Autodesk Inventor part; units mm, degrees
ref_plane "YZ Plane" through (0, 0, 0) normal (1, 0, 0) x (0, 1, 0)
ref_plane "XZ Plane" through (0, 0, 0) normal (0, 1, 0) x (-1, 0, 0)
ref_plane "XY Plane" through (0, 0, 0) normal (0, 0, 1) x (1, 0, 0)
sketch "C12,5-5, 470uF_126" plane through (0, 0, 0) normal (0, 0, 1) x (1, 0, 0)
  line L0 (0.9403, 6.3386) -> (1.557, 6.216)
  line L1 (1.557, 6.216) -> (2.1588, 6.0334)
  line L2 (2.1588, 6.0334) -> (2.7398, 5.7928)
  line L3 (2.7398, 5.7928) -> (3.2944, 5.4963)
  line L4 (3.2944, 5.4963) -> (3.8172, 5.147)
  line L5 (3.8172, 5.147) -> (4.3033, 4.748)
  line L6 (4.3033, 4.748) -> (4.748, 4.3034)
  line L7 (4.748, 4.3034) -> (5.147, 3.8172)
  line L8 (5.147, 3.8172) -> (5.4963, 3.2944)
  line L9 (5.4963, 3.2944) -> (5.7928, 2.7398)
  line L10 (5.7928, 2.7398) -> (6.0334, 2.1588)
  line L11 (6.0334, 2.1588) -> (6.216, 1.557)
  line L12 (6.216, 1.557) -> (6.3386, 0.9403)
  line L13 (6.3386, 0.9403) -> (6.4003, 0.3144)
  line L14 (6.4003, 0.3144) -> (6.4003, 0)
  line L15 (6.4003, 0) -> (6.4003, -0.3144)
  line L16 (6.4003, -0.3144) -> (6.3386, -0.9403)
  line L17 (6.3386, -0.9403) -> (6.216, -1.557)
  line L18 (6.216, -1.557) -> (6.0334, -2.1588)
  line L19 (6.0334, -2.1588) -> (5.7928, -2.7398)
  line L20 (5.7928, -2.7398) -> (5.4963, -3.2944)
  line L21 (5.4963, -3.2944) -> (5.147, -3.8172)
  line L22 (5.147, -3.8172) -> (4.748, -4.3033)
  line L23 (4.748, -4.3033) -> (4.3033, -4.748)
  line L24 (4.3033, -4.748) -> (3.8172, -5.147)
  line L25 (3.8172, -5.147) -> (3.2944, -5.4963)
  line L26 (3.2944, -5.4963) -> (2.7398, -5.7928)
  line L27 (2.7398, -5.7928) -> (2.1588, -6.0334)
  line L28 (2.1588, -6.0334) -> (1.557, -6.216)
  line L29 (1.557, -6.216) -> (0.9403, -6.3386)
  line L30 (0.9403, -6.3386) -> (0.3144, -6.4003)
  line L31 (0.3144, -6.4003) -> (-0.3144, -6.4003)
  line L32 (-0.3144, -6.4003) -> (-0.9403, -6.3386)
  line L33 (-0.9403, -6.3386) -> (-1.557, -6.216)
  line L34 (-1.557, -6.216) -> (-2.1588, -6.0334)
  line L35 (-2.1588, -6.0334) -> (-2.7398, -5.7928)
  line L36 (-2.7398, -5.7928) -> (-3.2944, -5.4963)
  line L37 (-3.2944, -5.4963) -> (-3.8172, -5.147)
  line L38 (-3.8172, -5.147) -> (-4.3034, -4.748)
  line L39 (-4.3034, -4.748) -> (-4.748, -4.3033)
  line L40 (-4.748, -4.3033) -> (-5.147, -3.8172)
  line L41 (-5.147, -3.8172) -> (-5.4963, -3.2944)
  line L42 (-5.4963, -3.2944) -> (-5.7928, -2.7398)
  line L43 (-5.7928, -2.7398) -> (-6.0334, -2.1588)
  line L44 (-6.0334, -2.1588) -> (-6.216, -1.557)
  line L45 (-6.216, -1.557) -> (-6.3386, -0.9403)
  line L46 (-6.3386, -0.9403) -> (-6.4003, -0.3144)
  line L47 (-6.4003, -0.3144) -> (-6.4003, 0)
  line L48 (-6.4003, 0) -> (-6.4003, 0.3144)
  line L49 (-6.4003, 0.3144) -> (-6.3386, 0.9403)
  line L50 (-6.3386, 0.9403) -> (-6.216, 1.557)
  line L51 (-6.216, 1.557) -> (-6.0334, 2.1588)
  line L52 (-6.0334, 2.1588) -> (-5.7928, 2.7398)
  line L53 (-5.7928, 2.7398) -> (-5.4963, 3.2944)
  line L54 (-5.4963, 3.2944) -> (-5.147, 3.8172)
  line L55 (-5.147, 3.8172) -> (-4.748, 4.3034)
  line L56 (-4.748, 4.3034) -> (-4.3034, 4.748)
  line L57 (-4.3034, 4.748) -> (-3.8172, 5.147)
  line L58 (-3.8172, 5.147) -> (-3.2944, 5.4963)
  line L59 (-3.2944, 5.4963) -> (-2.7398, 5.7928)
  line L60 (-2.7398, 5.7928) -> (-2.1588, 6.0334)
  line L61 (-2.1588, 6.0334) -> (-1.557, 6.216)
  line L62 (-1.557, 6.216) -> (-0.9403, 6.3386)
  line L63 (-0.9403, 6.3386) -> (-0.3144, 6.4003)
  line L64 (-0.3144, 6.4003) -> (0.3144, 6.4003)
  line L65 (0.3144, 6.4003) -> (0.9403, 6.3386)
extrude "Extrusion1" add sketch "C12,5-5, 470uF_126" along normal blind 20
properties part number "470uF"
Could you check a few things on this model? Use its own coordinates, in mm. Give positions to 0.01 mm unless a question says otherwise; leave off trailing zeros. Write each loop counter-clockwise with the first axis right and the second up, starting at its lowest first coordinate (ties: lowest second). Pieces come first, ordered by that corner, then holes. Notation, with made-up numbers: (-17.5, -32.5) -> (-2.5, -32.5) arc R36 cw to (-2.5, 5.5) -> close; hole circle Ø6 at (21, -9.5). An arc over 180 degrees is marked (long way). Write each question's results on one line, items separated by ' | '. Start each with the question number.
Q1. Suppose I cut it at A-A, the plane x = 2.5. List the corners of the cut face in (y, z) for me, and give its area (3 significant figures).
Q2. I need wall thicknesses on probe 1 along Y at (x, z) = (2.5, 10.25); probe 2 along X at (y, z) = (3, 17); probe 3 along X at (y, z) = (-5.25, 9.25). Which ranges of each line are inside material? Lowest first, please.
Q3. I'm going to push flat-ended pins straight in: pin 1 Ø1.5 at (x, z) = (-2.5, 3) entering from +Y; pin 2 Ø5 at (x, z) = (3, 4.5) entering from -Y; pin 3 Ø5 at (y, z) = (3, 10.5) entering from +X. Where does each tip first touch, or does it pass through?
Outcome:
1) outline: (-5.89, 0) -> (5.89, 0) -> (5.89, 20) -> (-5.89, 20) -> close | area: 236 mm2
2) probe 1: -5.89 to 5.89 | probe 2: -5.65 to 5.65 | probe 3: -3.66 to 3.66
3) pin 1: y = 6.16 | pin 2: y = -6.38 | pin 3: x = 6.38
